Geometry check sheet. Reference: the model listing, model coordinates, mm. A direction names the side the tool comes from. Coordinates: 2 decimals unless noted, no trailing zeros. Write each loop counter-clockwise with the first axis right and the second up, starting at its lowest first coordinate (ties: lowest second). Pieces come first, ordered by that corner, then holes.
from build123d import *

# Parameters (mm, degrees)
SKETCH4_W                 = 53.34
SKETCH4_H                 = 53.34
BOSS_EXTRUDE1_DEPTH       = 12.7
CUT_EXTRUDE1_DEPTH        = 11.43
F_4_40_TAPPED_HOLE1_D     = 2.2606
F_4_40_TAPPED_HOLE1_DEPTH = 11.43
SKETCH5_W                 = 50.8
SKETCH5_H                 = 50.8
CUT_EXTRUDE2_DEPTH        = 1.27
FILLET1_R                 = 1.27


with BuildPart() as part:
    # Sketch4 → Boss-Extrude1 (new body)
    with BuildSketch(Plane(origin=(0, 0, 0), x_dir=(1, 0, 0), z_dir=(0, 1, 0))):
        with Locations((25.4, 25.4)):
            Rectangle(SKETCH4_W, SKETCH4_H)
    extrude(amount=-BOSS_EXTRUDE1_DEPTH)

    # Sketch3 → Cut-Extrude1 (cut)
    with BuildSketch(Plane(origin=(0, 0, 0), x_dir=(1, 0, 0), z_dir=(0, 1, 0))):
        with BuildLine():
            Line((5.08, 0), (45.72, 0))
            ThreePointArc((45.72, 0), (46.618025612, 0.371974388), (46.99, 1.27))
            Line((46.99, 1.27), (46.99, 2.54))
            ThreePointArc((46.99, 2.54), (47.361974388, 3.438025612), (48.26, 3.81))
            Line((48.26, 3.81), (49.53, 3.81))
            ThreePointArc((49.53, 3.81), (50.428025612, 4.181974388), (50.8, 5.08))
            Line((50.8, 5.08), (50.8, 45.72))
            ThreePointArc((50.8, 45.72), (50.428025612, 46.618025612), (49.53, 46.99))
            Line((49.53, 46.99), (48.26, 46.99))
            ThreePointArc((48.26, 46.99), (47.361974388, 47.361974388), (46.99, 48.26))
            Line((46.99, 48.26), (46.99, 49.53))
            ThreePointArc((46.99, 49.53), (46.618025612, 50.428025612), (45.72, 50.8))
            Line((45.72, 50.8), (5.08, 50.8))
            ThreePointArc((5.08, 50.8), (4.181974388, 50.428025612), (3.81, 49.53))
            Line((3.81, 49.53), (3.81, 48.26))
            ThreePointArc((3.81, 48.26), (3.438025612, 47.361974388), (2.54, 46.99))
            Line((2.54, 46.99), (1.27, 46.99))
            ThreePointArc((1.27, 46.99), (0.371974388, 46.618025612), (0, 45.72))
            Line((0, 45.72), (0, 5.08))
            ThreePointArc((0, 5.08), (0.371974388, 4.181974388), (1.27, 3.81))
            Line((1.27, 3.81), (2.54, 3.81))
            ThreePointArc((2.54, 3.81), (3.438025612, 3.438025612), (3.81, 2.54))
            Line((3.81, 2.54), (3.81, 1.27))
            ThreePointArc((3.81, 1.27), (4.181974388, 0.371974388), (5.08, 0))
        make_face()
    extrude(amount=-CUT_EXTRUDE1_DEPTH, mode=Mode.SUBTRACT)

    # #4-40 Tapped Hole1
    with Locations(Plane(origin=(0, 0, 0), x_dir=(1, 0, 0), z_dir=(0, 1, 0))):
        with Locations((1.905, 48.895), (48.895, 48.895), (1.905, 1.905), (48.895, 1.905)):
            Hole(F_4_40_TAPPED_HOLE1_D / 2, depth=F_4_40_TAPPED_HOLE1_DEPTH)

    # Sketch5 → Cut-Extrude2 (cut)
    with BuildSketch(Plane(origin=(0, 0, 0), x_dir=(1, 0, 0), z_dir=(0, 1, 0))):
        with Locations((25.4, 25.4)):
            Rectangle(SKETCH5_W, SKETCH5_H)
    extrude(amount=-CUT_EXTRUDE2_DEPTH, mode=Mode.SUBTRACT)

    # Fillet1
    fillet1_edges = [part.edges().sort_by_distance(p)[0] for p in [
        (-1.27, -6.35, -52.07),
        (52.07, -6.35, -52.07),
        (52.07, -6.35, 1.27),
        (-1.27, -6.35, 1.27),
    ]]
    fillet(fillet1_edges, radius=FILLET1_R)


solid = part.part
1. Sectioned sample at B-B, the plane z = -27. Record the boundary of the cut face in (x, y).
Computed values:
outline: (-1.27, -12.7) - (52.07, -12.7) - (52.07, 0) - (50.8, 0) - (50.8, -11.43) - (0, -11.43) - (0, 0) - (-1.27, 0) - close
2. Access from +Z, -Z, +X, -X, +Y, -Y to the whole of each face (thin tool, end or side, straight path). Record for faces 1 (the flat face through (49, -11.43, -2)), 2 (the flat face through (25, -6, -52.07)).
Computed values:
face 1: +Y
face 2: -Z, +X, -X, +Y, -Y
3. Sectioned sample at C-C, the plane y = -7. Give the number of separate pieces and of enclosed holes in the cut face, and give its area (3 significant figures).
Computed values:
separate pieces: 1
enclosed holes: 5
area: 307 mm2
4. Thickness scan on line 1 along Z through (x, y) = (49, -10); line 2 along X through (y, z) = (-7.75, -2); line 3 along Z through (x, y) = (9.5, -2.5). Record the ranges inside material, lowest first.
Computed values:
line 1: z = -52.07 to -50.02, -47.77 to -46.99, -3.81 to -3.03, -0.78 to 1.27
line 2: x = -1.27 to 0.78, 3.03 to 3.81, 46.99 to 47.77, 50.02 to 52.07
line 3: z = -52.07 to -50.8, 0 to 1.27
5. Draft check along Z on faces 3 (the cylindrical face through (51.708, -6.439, 0.888)), 4 (the flat face through (49, -6, -3.81)), 5 (the cylindrical face through (48.29, -6.42, -49.85)), 6 (the flat face through (25, -12.7, -26)). Enter one of: released by +Z, released by -Z, zero draft, split by the parting line, or undercut.
Computed values:
face 3: released by +Z
face 4: undercut
face 5: undercut
face 6: zero draft
6. Gauge pin test, flat ends, axial feed: pin 1 Ø1.4 at (x, z) = (1.905, -48.895) entering from +Y; pin 2 Ø2.5 at (x, z) = (49, -48.5) entering from +Y. Record the tip position at first contact, or that the pin passes through.
Computed values:
pin 1: stops at y = -11.43
pin 2: stops at y = -1.27
7. Sectioned sample at A-A, the plane x = 29.5. Record the boundary of the cut face in (y, z).
Computed values:
outline: (-12.7, -52.07) - (0, -52.07) - (0, -50.8) - (-11.43, -50.8) - (-11.43, 0) - (0, 0) - (0, 1.27) - (-12.7, 1.27) - close
